from build123d import *

# Parameters (mm, degrees)
SKETCH1_W               = 50.8
SKETCH1_H               = 39.395334333
SKETCH1_R               = 2.75
SKETCH1_R_2             = 7.747
BOSS_EXTRUDE1_DEPTH     = 38.35
CUT_EXTRUDE1_DEPTH      = 100.182747326
CUT_EXTRUDE1_DEPTH_BACK = 100.182747326
SKETCH2_W               = 1.27
SKETCH2_H               = 7
CUT_EXTRUDE2_DEPTH      = 71.04748878
CUT_EXTRUDE2_DEPTH_BACK = 71.04748878
SKETCH3_R               = 1
FILLET1_R               = 6.35


with BuildPart() as part:
    # Sketch1 → Boss-Extrude1 (new body)
    with BuildSketch(Plane.XY):
        with Locations((-57.15, 9.547643302)):
            Rectangle(SKETCH1_W, SKETCH1_H)
        with Locations(Location((-57.15, 23.269976885, 0), (0, 0, 180))):
            Circle(SKETCH1_R, mode=Mode.SUBTRACT)
        with Locations(Location((-57.15, -4.174690282, 0), (0, 0, 180))):
            Circle(SKETCH1_R, mode=Mode.SUBTRACT)
        with Locations(Location((-57.15, 9.547643302, 0), (0, 0, 180))):
            Circle(SKETCH1_R_2, mode=Mode.SUBTRACT)
    extrude(amount=BOSS_EXTRUDE1_DEPTH)

    # Sketch2 → Cut-Extrude1 (cut, two sides: drawn at the far end of the back side and taken through both)
    with BuildSketch(Plane(origin=(0, -10.150023865, 0), x_dir=(-1, 0, 0), z_dir=(0, -1, 0)).offset(-CUT_EXTRUDE1_DEPTH_BACK)):
        with Locations((72.6, -17.65)):
            Rectangle(SKETCH2_W, SKETCH2_H)
        with Locations((41.7, -27.05)):
            Rectangle(SKETCH2_W, SKETCH2_H)
        with Locations((41.7, -17.65)):
            Rectangle(SKETCH2_W, SKETCH2_H)
        with Locations((72.6, -27.05)):
            Rectangle(SKETCH2_W, SKETCH2_H)
    extrude(amount=CUT_EXTRUDE1_DEPTH + CUT_EXTRUDE1_DEPTH_BACK, mode=Mode.SUBTRACT)

    # Sketch3 → Cut-Extrude2 (cut, two sides: drawn at the far end of the back side and taken through both)
    with BuildSketch(Plane(origin=(-31.75, 0, 0), x_dir=(0, 0, -1), z_dir=(1, 0, 0)).offset(-CUT_EXTRUDE2_DEPTH_BACK)):
        with Locations((-17.65, 9.547643302)):
            Circle(SKETCH3_R)
        with Locations(Location((-27.05, 9.547643302, 0), (0, 0, 90))):
            Circle(SKETCH3_R)
    extrude(amount=CUT_EXTRUDE2_DEPTH + CUT_EXTRUDE2_DEPTH_BACK, mode=Mode.SUBTRACT)

    # Fillet1
    fillet1_edges = [part.edges().sort_by_distance(p)[0] for p in [
        (-31.75, -10.150023865, 19.175),
        (-82.55, -10.150023865, 19.175),
        (-82.55, 29.245310468, 19.175),
        (-31.75, 29.245310468, 19.175),
    ]]
    fillet(fillet1_edges, radius=FILLET1_R)


solid = part.part
Verification items for the finished model (mm, model axes). A direction names the side the tool comes from. Round coordinates to 2 decimals unless told otherwise and drop trailing zeros. Loops run counter-clockwise (first coordinate to the right, second up) from the corner with the lowest first, then second, coordinate; pieces in that order, holes last. Notation, with made-up numbers: (69.5, 80) - (104.5, 80) arc R23 cw to (104.5, 105) - close; hole circle Ø4 at (50, 43.5). An arc over 180 degrees is marked (long way). Write item = value, one per line.
Q1. Sectioned sample at A-A on x = -57.15. Record the boundary of the cut face in (y, z).
Here are the results:
outline = (-10.15, 0) - (-6.92, 0) - (-6.92, 38.35) - (-10.15, 38.35) - close; (-1.42, 0) - (1.8, 0) - (1.8, 38.35) - (-1.42, 38.35) - close; (17.29, 0) - (20.52, 0) - (20.52, 38.35) - (17.29, 38.35) - close; (26.02, 0) - (29.25, 0) - (29.25, 38.35) - (26.02, 38.35) - close
Q2. Sectioned sample at B-B on y = 14. Record the boundary of the cut face in (x, z) (3 decimals).
Here are the results:
outline = (-82.55, 0) - (-63.49, 0) - (-63.49, 38.35) - (-82.55, 38.35) - close; (-50.81, 0) - (-31.75, 0) - (-31.75, 38.35) - (-50.81, 38.35) - close; hole (-73.235, 14.15) - (-71.965, 14.15) - (-71.965, 21.15) - (-73.235, 21.15) - close; hole (-73.235, 23.55) - (-71.965, 23.55) - (-71.965, 30.55) - (-73.235, 30.55) - close; hole (-42.335, 14.15) - (-41.065, 14.15) - (-41.065, 21.15) - (-42.335, 21.15) - close; hole (-42.335, 23.55) - (-41.065, 23.55) - (-41.065, 30.55) - (-42.335, 30.55) - close
Q3. Mould release check, pull along Z, two halves, no side actions. Record for faces 1 (the flat face through (-58, 19, 38.35)), 2 (the cylindrical face through (-36.473, 9.848, 16.696)), 3 (the cylindrical face through (-33.66, 27.435, 19.443)): +Z half, -Z half, draft (parallel to the pull), parting line (faces both ways), or undercut.
Here are the results:
face_1 = +Z half
face_2 = undercut
face_3 = draft
Q4. Sectioned sample at C-C on z = 29.5. Record the boundary of the cut face in (x, y) (3 decimals).
Here are the results:
outline = (-82.55, -3.8) arc R6.35 ccw to (-76.2, -10.15) - (-73.235, -10.15) - (-73.235, 29.245) - (-76.2, 29.245) arc R6.35 ccw to (-82.55, 22.895) - close; (-71.965, -10.15) - (-42.335, -10.15) - (-42.335, 29.245) - (-71.965, 29.245) - close; (-41.065, -10.15) - (-38.1, -10.15) arc R6.35 ccw to (-31.75, -3.8) - (-31.75, 22.895) arc R6.35 ccw to (-38.1, 29.245) - (-41.065, 29.245) - close; hole circle Ø15.494 at (-57.15, 9.548); hole circle Ø5.5 at (-57.15, -4.175); hole circle Ø5.5 at (-57.15, 23.27)
Q5. Material ranges on L1, parallel to X at y = 18, z = 18 (3 decimals); L2, parallel to Z at x = -72, y = 24; L3, parallel to X at y = 14, z = 24 (3 decimals), recorded low to high.
Here are the results:
L1 = -82.55 to -73.235, -71.965 to -42.335, -41.065 to -31.75
L2 = 0 to 14.15, 21.15 to 23.55, 30.55 to 38.35
L3 = -82.55 to -73.235, -71.965 to -63.49, -50.81 to -42.335, -41.065 to -31.75
Q6. Tool access check on faces 4 (the flat face through (-42.335, 10, 16)), 5 (the cylindrical face through (-33.66, -8.34, 19.44)). Record the directions out of +Z, -Z, +X, -X, +Y, -Y that give a thin tool (end or side, any length) a straight path to the whole face; none if there is none.
Here are the results:
face_4 = +Y, -Y
face_5 = +Z, -Z, +X, -Y
Q7. Sectioned sample at D-D on y = 0.5. Record the boundary of the cut face in (x, z) (3 decimals).
Here are the results:
outline = (-82.55, 0) - (-31.75, 0) - (-31.75, 38.35) - (-82.55, 38.35) - close; hole (-73.235, 14.15) - (-71.965, 14.15) - (-71.965, 21.15) - (-73.235, 21.15) - close; hole (-73.235, 23.55) - (-71.965, 23.55) - (-71.965, 30.55) - (-73.235, 30.55) - close; hole (-42.335, 14.15) - (-41.065, 14.15) - (-41.065, 21.15) - (-42.335, 21.15) - close; hole (-42.335, 23.55) - (-41.065, 23.55) - (-41.065, 30.55) - (-42.335, 30.55) - close
